from build123d import *

# Parameters (mm, degrees)
SKETCH1_W           = 100
SKETCH1_H           = 52
SKETCH1_R           = 2.5
SKETCH1_R_2         = 2
BOSS_EXTRUDE1_DEPTH = 3
FILLET1_R           = 15
FILLET2_R           = 7


with BuildPart() as part:
    # Sketch1 → Boss-Extrude1 (new body)
    with BuildSketch(Plane(origin=(0, 0, 0), x_dir=(1, 0, 0), z_dir=(0, 1, 0))):
        Rectangle(SKETCH1_W, SKETCH1_H)
        with Locations((41, 0)):
            Circle(SKETCH1_R, mode=Mode.SUBTRACT)
        with Locations((-41, 19)):
            Circle(SKETCH1_R, mode=Mode.SUBTRACT)
        with Locations((-41, -19)):
            Circle(SKETCH1_R, mode=Mode.SUBTRACT)
        with Locations((-31, 21.2)):
            Circle(SKETCH1_R_2, mode=Mode.SUBTRACT)
        with Locations((-31, 7.7)):
            Circle(SKETCH1_R_2, mode=Mode.SUBTRACT)
    extrude(amount=BOSS_EXTRUDE1_DEPTH)

    # Fillet1
    fillet1_edges = [part.edges().sort_by_distance(p)[0] for p in [
        (50, 1.5, 26),
        (50, 1.5, -26),
    ]]
    fillet(fillet1_edges, radius=FILLET1_R)

    # Fillet2
    fillet2_edges = [part.edges().sort_by_distance(p)[0] for p in [
        (-50, 1.5, 26),
        (-50, 1.5, -26),
    ]]
    fillet(fillet2_edges, radius=FILLET2_R)


solid = part.part
Could you check a few things on this model? Use its own coordinates, in mm. Give positions to 0.01 mm unless a question says otherwise; leave off trailing zeros. Order: outer loops, then holes, each group sorted by start corner. A loop starts at its lowest first (then second) coordinate and runs counter-clockwise, first axis right, second up. Notation, with made-up numbers: (85, -9.75) - (133, -9.75) arc R36 ccw to (133, 24.25) - close; hole circle Ø11 at (65.5, 10). An arc over 180 degrees is marked (long way). Return JSON: item names as keys, results as strings. Group by question number.
Q1. Suppose I cut it at A-A, the plane x = -31. Please give me the cut outline in (y, z).
Q2. Will these pins go through, and if not, where does the flat tip stop? pin 1 Ø3.5 at (x, z) = (-31, -7.7) entering from +Y; pin 2 Ø1 at (x, z) = (22, 6) entering from -Y.
Q3. Suppose I cut it at C-C, the plane z = -7.7. Please give me the cut outline in (x, y).
Q4. Thinking about a two-plate mould opening in Z: for faces 1 (the face through (50, 1, 0)), 2 (the face through (-5, 1, 26)), 3 (the face through (-38.615, 1.479, 18.249)), which applies, pulls with the +Z half, pulls with the -Z half, needs draft (parallel to the pull), parting line crosses it, or undercut?
Q5. Suppose I cut it at D-D, the plane x = 42.5. Please give me the cut outline in (y, z).
Q6. Please list where these lines run through material, in increasing order: line 1 along Z through (x, y) = (-31, 1.9); line 2 along Z through (x, y) = (-41, 1.9); line 3 along X through (y, z) = (0.7, -21.2). Write a range as [from, to].
Q7. Suppose I cut it at B-B, the plane y = 1.85. Please give me the cut outline in (x, z).
Resolved:
{
 "1": {"outline": "(0, -26) - (3, -26) - (3, -23.2) - (0, -23.2) - close; (0, -19.2) - (3, -19.2) - (3, -9.7) - (0, -9.7) - close; (0, -5.7) - (3, -5.7) - (3, 26) - (0, 26) - close"},
 "2": {"pin 1": "passes through", "pin 2": "stops at y = 0"},
 "3": {"outline": "(-50, 0) - (-33, 0) - (-33, 3) - (-50, 3) - close; (-29, 0) - (50, 0) - (50, 3) - (-29, 3) - close"},
 "4": {"face 1": "needs draft", "face 2": "pulls with the +Z half", "face 3": "undercut"},
 "5": {"outline": "(0, -23.99) - (3, -23.99) - (3, -2) - (0, -2) - close; (0, 2) - (3, 2) - (3, 23.99) - (0, 23.99) - close"},
 "6": {"line 1": "z = [-26, -23.2], [-19.2, -9.7], [-5.7, 26]", "line 2": "z = [-26, -21.5], [-16.5, 16.5], [21.5, 26]", "line 3": "x = [-49.65, -42.19], [-39.81, -33], [-29, 46]"},
 "7": {"outline": "(-50, -19) arc R7 ccw to (-43, -26) - (35, -26) arc R15 ccw to (50, -11) - (50, 11) arc R15 ccw to (35, 26) - (-43, 26) arc R7 ccw to (-50, 19) - close; hole circle Ø5 at (-41, -19); hole circle Ø5 at (-41, 19); hole circle Ø4 at (-31, -21.2); hole circle Ø4 at (-31, -7.7); hole circle Ø5 at (41, 0)"}
}
